Read the model definition and answer for the solid it produces. Units are mm, in the model's axes. A direction names the side the tool comes from. Round coordinates to 2 decimals unless told otherwise and drop trailing zeros. Order: outer loops, then holes, each group sorted by start corner. A loop starts at its lowest first (then second) coordinate and runs counter-clockwise, first axis right, second up. Notation, with made-up numbers: M -34,19 L -25,19 A21 cw -25,28 Z; hole C 39,14.25 d11. An arc over 180 degrees is marked long. Answer as CSV lines item,"result".
```python
from build123d import *

# Parameters (mm, degrees)
SALIENTE_EXTRUIR1_DEPTH = 30
CROQUIS2_R              = 1.5
CORTAR_EXTRUIR1_DEPTH   = 30
CROQUIS3_R              = 1.5
CORTAR_EXTRUIR2_DEPTH   = 30


with BuildPart() as part:
    # Croquis1 → Saliente-Extruir1 (new body)
    with BuildSketch(Plane.XY):
        Polygon((0, 0), (20, 0), (20, 20), (25, 20), (25, -5), (0, -5), align=None)
    extrude(amount=SALIENTE_EXTRUIR1_DEPTH)

    # Croquis2 → Cortar-Extruir1 (cut)
    with BuildSketch(Plane(origin=(25, 0, 0), x_dir=(0, 0, -1), z_dir=(1, 0, 0))):
        with Locations((-25, 7)):
            Circle(CROQUIS2_R)
        with Locations((-5, 7)):
            Circle(CROQUIS2_R)
    extrude(amount=-CORTAR_EXTRUIR1_DEPTH, mode=Mode.SUBTRACT)

    # Croquis3 → Cortar-Extruir2 (cut)
    with BuildSketch(Plane.XZ.offset(5)):
        with Locations((5, 5)):
            Circle(CROQUIS3_R)
        with Locations((5, 25)):
            Circle(CROQUIS3_R)
    extrude(amount=-CORTAR_EXTRUIR2_DEPTH, mode=Mode.SUBTRACT)


solid = part.part
```
Item 1: Determine the mould class of faces 3 (the face through (22.535, 5.536, 5.325)), 4 (the face through (4.805, -2.535, 26.487)), 5 (the face through (20, 10, 15)) for opening direction X: +X half, -X half, draft (parallel to the pull), parting line (faces both ways), or undercut.
Ans:
face 3,"draft"
face 4,"undercut"
face 5,"-X half"
Item 2: A cutting plane is placed at C-C, the plane y = -2.25. Determine the outline of the cut face in (x, z).
Ans:
outline,"M 0,0 L 25,0 L 25,30 L 0,30 Z; hole C 5,5 d3; hole C 5,25 d3"
Item 3: A cutting plane is placed at A-A, the plane x = 5. Determine the outline of the cut face in (y, z).
Ans:
outline,"M -5,0 L 0,0 L 0,3.5 L -5,3.5 Z; M -5,6.5 L 0,6.5 L 0,23.5 L -5,23.5 Z; M -5,26.5 L 0,26.5 L 0,30 L -5,30 Z"
Item 4: A cutting plane is placed at D-D, the plane z = 10. Determine the outline of the cut face in (x, y).
Ans:
outline,"M 0,-5 L 25,-5 L 25,20 L 20,20 L 20,0 L 0,0 Z"
Item 5: A cutting plane is placed at B-B, the plane z = 5. Determine the outline of the cut face in (x, y).
Ans:
outline,"M 0,-5 L 3.5,-5 L 3.5,0 L 0,0 Z; M 6.5,-5 L 25,-5 L 25,5.5 L 20,5.5 L 20,0 L 6.5,0 Z; M 20,8.5 L 25,8.5 L 25,20 L 20,20 Z"
Item 6: Flat-ended cylindrical pins translate along their axes: pin 1 (5 mm diameter, centred on x = 22, y = 4, fed in from -Z); pin 2 (6 mm diameter, centred on y = 9, z = 9, fed in from -X); pin 3 (5 mm diameter, centred on x = 5, z = 25, fed in from +Y). Find the tip coordinate at first contact, or state that the pin passes through.
Ans:
pin 1,"z = 0"
pin 2,"x = 20"
pin 3,"y = 0"
Item 7: Find the intervals of material crossed by probe 1 along Y at (x, z) = (3.5, 1.5); probe 2 along Y at (x, z) = (21.8, 25); probe 3 along X at (y, z) = (9.25, 26), in increasing order. Write a range as [from, to].
Ans:
probe 1,"[-5, 0]"
probe 2,"[-5, 5.5], [8.5, 20]"
probe 3,"[20, 25]"
Item 8: A tool of negligible diameter and unlimited length cuts with its end or side. For faces 1 (the face through (22.54, 7.07, 26.5)), 2 (the face through (10, 0, 15)), from which of +Z, -Z, +X, -X, +Y, -Y can it reach the whole face along a straight path? Write none if from no direction.
Ans:
face 1,"+X, -X"
face 2,"+Z, -Z, -X, +Y"
